Here's how the part is built. I have some questions about the finished solid (model axes, mm). Give positions to 0.01 mm unless a question says otherwise; leave off trailing zeros. Loops run counter-clockwise (first coordinate to the right, second up) from the corner with the lowest first, then second, coordinate; pieces in that order, holes last. Notation, with made-up numbers: (21.5, -4.75) - (45.5, -4.75) arc R24 ccw to (45.5, 10.25) - close; hole circle Ø6 at (-33, 0.5). An arc over 180 degrees is marked (long way). Use a Markdown table: item, result.
from build123d import *

# Parameters (mm, degrees)
SKETCH1_W                = 115
SKETCH1_H                = 36.5
BOSS_EXTRUDE1_DEPTH      = 1
BOSS_EXTRUDE2_DEPTH      = 20
BOSS_EXTRUDE2_DEPTH_BACK = 1
SKETCH2_W                = 119
SKETCH2_H                = 40.5
SKETCH2_W_2              = 115
SKETCH2_H_2              = 36.5
SKETCH3_R                = 1.5
SKETCH3_W                = 6
SKETCH3_H                = 6
BOSS_EXTRUDE3_DEPTH      = 3
SKETCH4_R                = 1.5
SKETCH4_W                = 5.5
SKETCH4_H                = 6.495155074
BOSS_EXTRUDE4_DEPTH      = 8
SKETCH5_W                = 15
SKETCH5_H                = 10
CUT_EXTRUDE1_DEPTH       = 8
SKETCH6_W                = 46
SKETCH6_H                = 7.792677535
CUT_EXTRUDE2_DEPTH       = 8
SKETCH7_W                = 10.3
SKETCH7_H                = 10.3
CUT_EXTRUDE3_DEPTH       = 8
SKETCH8_W                = 15
SKETCH8_H                = 5
CUT_EXTRUDE4_DEPTH       = 8
SKETCH9_W                = 119
SKETCH9_H                = 40.5
SKETCH9_W_2              = 17
SKETCH9_H_2              = 17
SKETCH9_W_3              = 73
SKETCH9_H_3              = 26
BOSS_EXTRUDE5_DEPTH      = 3
SKETCH10_W               = 119
SKETCH10_H               = 40.5
SKETCH10_W_2             = 115
SKETCH10_H_2             = 36.5
CUT_EXTRUDE5_DEPTH       = 2


with BuildPart() as part:
    # Sketch1 → Boss-Extrude1 (new body)
    with BuildSketch(Plane(origin=(0, 0, 0), x_dir=(1, 0, 0), z_dir=(0, 1, 0))):
        Rectangle(SKETCH1_W, SKETCH1_H)
    extrude(amount=BOSS_EXTRUDE1_DEPTH)


with BuildPart() as body_2:
    # Sketch2 → Boss-Extrude2 (new, two sides: drawn at the far end of the back side and taken through both)
    with BuildSketch(Plane(origin=(0, 1, 0), x_dir=(1, 0, 0), z_dir=(0, 1, 0)).offset(-BOSS_EXTRUDE2_DEPTH_BACK)):
        Rectangle(SKETCH2_W, SKETCH2_H)
        Rectangle(SKETCH2_W_2, SKETCH2_H_2, mode=Mode.SUBTRACT)
    extrude(amount=BOSS_EXTRUDE2_DEPTH + BOSS_EXTRUDE2_DEPTH_BACK)

    # Intersect1: read off the stored shape, not the designer's step
    # Intersect1: union part
    add(part.part)

    # Sketch3 → Boss-Extrude3 (add)
    # profile 1 of 4: a face of its own
    with BuildSketch(Plane(origin=(0, 1, 0), x_dir=(1, 0, 0), z_dir=(0, 1, 0))):
        Polygon((-51.5, 7.25), (-51.5, 13.25), (-54, 13.25), (-57.5, 13.25), (-57.5, 9.75), (-57.5, 7.25), align=None)
        with Locations(Location((-54, 9.75, 0), (0, 0, 270))):
            Circle(SKETCH3_R, mode=Mode.SUBTRACT)
    # profile 2 of 4: a face of its own
    with BuildSketch(Plane(origin=(0, 1, 0), x_dir=(1, 0, 0), z_dir=(0, 1, 0))):
        with Locations((-25.5, 10.25)):
            Rectangle(SKETCH3_W, SKETCH3_H)
        with Locations(Location((-26, 9.75, 0), (0, 0, 90))):
            Circle(SKETCH3_R, mode=Mode.SUBTRACT)
    # profile 3 of 4: a face of its own
    with BuildSketch(Plane(origin=(0, 1, 0), x_dir=(1, 0, 0), z_dir=(0, 1, 0))):
        with Locations((-25.5, -10.25)):
            Rectangle(SKETCH3_W, SKETCH3_H)
        with Locations(Location((-26, -9.75, 0), (0, 0, 270))):
            Circle(SKETCH3_R, mode=Mode.SUBTRACT)
    # profile 4 of 4: a face of its own
    with BuildSketch(Plane(origin=(0, 1, 0), x_dir=(1, 0, 0), z_dir=(0, 1, 0))):
        with Locations((-54.5, -10.25)):
            Rectangle(SKETCH3_W, SKETCH3_H)
        with Locations(Location((-54, -9.75, 0), (0, 0, 90))):
            Circle(SKETCH3_R, mode=Mode.SUBTRACT)
    extrude(amount=BOSS_EXTRUDE3_DEPTH)

    # Sketch4 → Boss-Extrude4 (add)
    # profile 1 of 4: a face of its own
    with BuildSketch(Plane(origin=(0, 1, 0), x_dir=(1, 0, 0), z_dir=(0, 1, 0))):
        Polygon((-22.5, 13.25), (-22.5, 11.754844926), (-17, 11.754844926), (-17, 18.25), (-20, 18.25), (-22.5, 18.25), (-22.5, 15.25), align=None)
        with Locations(Location((-20, 15.25, 0), (0, 0, 270))):
            Circle(SKETCH4_R, mode=Mode.SUBTRACT)
    # profile 2 of 4: a face of its own
    with BuildSketch(Plane(origin=(0, 1, 0), x_dir=(1, 0, 0), z_dir=(0, 1, 0))):
        with Locations((-19.75, -15.002422463)):
            Rectangle(SKETCH4_W, SKETCH4_H)
        with Locations(Location((-20, -15.25, 0), (0, 0, 90))):
            Circle(SKETCH4_R, mode=Mode.SUBTRACT)
    # profile 3 of 4: a face of its own
    with BuildSketch(Plane(origin=(0, 1, 0), x_dir=(1, 0, 0), z_dir=(0, 1, 0))):
        with Locations((54.75, -15.002422463)):
            Rectangle(SKETCH4_W, SKETCH4_H)
        with Locations(Location((55, -15.25, 0), (0, 0, 270))):
            Circle(SKETCH4_R, mode=Mode.SUBTRACT)
    # profile 4 of 4: a face of its own
    with BuildSketch(Plane(origin=(0, 1, 0), x_dir=(1, 0, 0), z_dir=(0, 1, 0))):
        with Locations((54.75, 15.002422463)):
            Rectangle(SKETCH4_W, SKETCH4_H)
        with Locations(Location((55, 15.25, 0), (0, 0, 90))):
            Circle(SKETCH4_R, mode=Mode.SUBTRACT)
    extrude(amount=BOSS_EXTRUDE4_DEPTH)

    # Sketch5 → Cut-Extrude1 (cut)
    with BuildSketch(Plane.ZY.offset(59.5)):
        with Locations((0, 11.525411997)):
            Rectangle(SKETCH5_W, SKETCH5_H)
    extrude(amount=-CUT_EXTRUDE1_DEPTH, mode=Mode.SUBTRACT)

    # Sketch6 → Cut-Extrude2 (cut)
    with BuildSketch(Plane(origin=(0, 0, -20.25), x_dir=(-1, 0, 0), z_dir=(0, 0, -1))):
        with Locations((-6.5, 11.396338768)):
            Rectangle(SKETCH6_W, SKETCH6_H)
    extrude(amount=-CUT_EXTRUDE2_DEPTH, mode=Mode.SUBTRACT)

    # Sketch7 → Cut-Extrude3 (cut)
    with BuildSketch(Plane.XY.offset(20.25)):
        with Locations((-49.05, 10.55)):
            Rectangle(SKETCH7_W, SKETCH7_H)
    extrude(amount=-CUT_EXTRUDE3_DEPTH, mode=Mode.SUBTRACT)

    # Sketch8 → Cut-Extrude4 (cut)
    with BuildSketch(Plane(origin=(0, 0, -20.25), x_dir=(-1, 0, 0), z_dir=(0, 0, -1))):
        with Locations((40.794043984, 3.5)):
            Rectangle(SKETCH8_W, SKETCH8_H)
    extrude(amount=-CUT_EXTRUDE4_DEPTH, mode=Mode.SUBTRACT)


with BuildPart() as body_2_2:
    # Sketch9 → Boss-Extrude5 (new body)
    with BuildSketch(Plane(origin=(0, 21, 0), x_dir=(1, 0, 0), z_dir=(0, 1, 0))):
        Rectangle(SKETCH9_W, SKETCH9_H)
        with Locations((-40, 1.75)):
            Rectangle(SKETCH9_W_2, SKETCH9_H_2, mode=Mode.SUBTRACT)
        with Locations((17.25, -0.25)):
            Rectangle(SKETCH9_W_3, SKETCH9_H_3, mode=Mode.SUBTRACT)
    extrude(amount=BOSS_EXTRUDE5_DEPTH)

    # Sketch10 → Cut-Extrude5 (cut)
    with BuildSketch(Plane.XZ.offset(-21)):
        Rectangle(SKETCH10_W, SKETCH10_H)
        Rectangle(SKETCH10_W_2, SKETCH10_H_2, mode=Mode.SUBTRACT)
    extrude(amount=-CUT_EXTRUDE5_DEPTH, mode=Mode.SUBTRACT)


solid = body_2_2.part
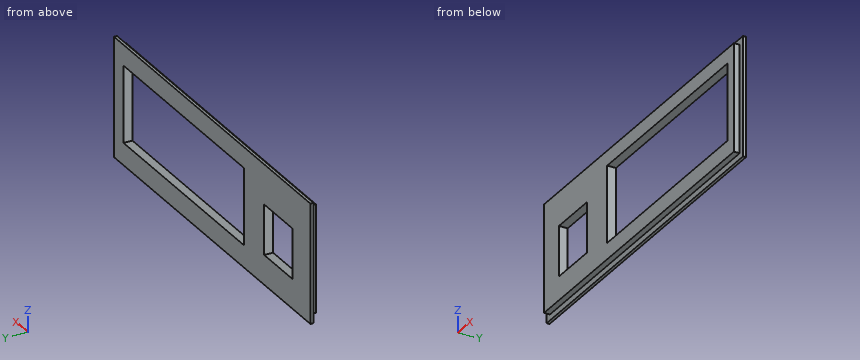
(1) Will these pins go through, and if not, where does the flat tip stop? pin 1 (1.6 mm diameter, centred on x = 12.5, y = 22, fed in from +Z); pin 2 (0.9 mm diameter, centred on x = 16, y = 22, fed in from -Z).
A:
| item | result |
|---|---|
| pin 1 | z = 18.25 |
| pin 2 | z = -18.25 |
(2) Suppose I cut it at D-D on y = 21.65. Write out the boundary of the cut face in (x, z), plus the area to 3 significant figures.
A:
| item | result |
|---|---|
| outline | (-57.5, -18.25) - (57.5, -18.25) - (57.5, 18.25) - (-57.5, 18.25) - close; hole (-48.5, -10.25) - (-31.5, -10.25) - (-31.5, 6.75) - (-48.5, 6.75) - close; hole (-19.25, -12.75) - (53.75, -12.75) - (53.75, 13.25) - (-19.25, 13.25) - close |
| area | 2,010 mm2 |
(3) If I drill on line 1 (X direction, y = 21.7, z = -1); line 2 (Z direction, x = 42, y = 22.45); line 3 (X direction, y = 21.9, z = 10), over which ranges is the centre line in solid material (lowest first)?
A:
| item | result |
|---|---|
| line 1 | -57.5 to -48.5, -31.5 to -19.25, 53.75 to 57.5 |
| line 2 | -18.25 to -12.75, 13.25 to 18.25 |
| line 3 | -57.5 to -19.25, 53.75 to 57.5 |
(4) Suppose I cut it at C-C on z = 4.5. Write out the boundary of the cut face in (x, y), plus the area to 3 significant figures.
A:
| item | result |
|---|---|
| outline | (-59.5, 23) - (-57.5, 23) - (-57.5, 21) - (-48.5, 21) - (-48.5, 24) - (-59.5, 24) - close; (-31.5, 21) - (-19.25, 21) - (-19.25, 24) - (-31.5, 24) - close; (53.75, 21) - (57.5, 21) - (57.5, 23) - (59.5, 23) - (59.5, 24) - (53.75, 24) - close |
| area | 79.0 mm2 |
(5) Suppose I cut it at A-A on z = 11.5. Write out the boundary of the cut face in (x, y), plus the area to 3 significant figures.
A:
| item | result |
|---|---|
| outline | (-59.5, 23) - (-57.5, 23) - (-57.5, 21) - (-19.25, 21) - (-19.25, 24) - (-59.5, 24) - close; (53.75, 21) - (57.5, 21) - (57.5, 23) - (59.5, 23) - (59.5, 24) - (53.75, 24) - close |
| area | 130 mm2 |
(6) Suppose I cut it at B-B on x = 32. Write out the boundary of the cut face in (y, z), plus the area to 3 significant figures.
A:
| item | result |
|---|---|
| outline | (21, -18.25) - (23, -18.25) - (23, -20.25) - (24, -20.25) - (24, -12.75) - (21, -12.75) - close; (21, 13.25) - (24, 13.25) - (24, 20.25) - (23, 20.25) - (23, 18.25) - (21, 18.25) - close |
| area | 35.5 mm2 |
